Autodesk Inventor part; units mm, degrees
ref_plane "YZ Plane" through (0, 0, 0) normal (1, 0, 0) x (0, 1, 0)
ref_plane "XZ Plane" through (0, 0, 0) normal (0, 1, 0) x (-1, 0, 0)
ref_plane "XY Plane" through (0, 0, 0) normal (0, 0, 1) x (1, 0, 0)
sketch "Sketch1" plane through (0, 0, 0) normal (0, 0, 1) x (1, 0, 0)
  circle A0 centre (16.975, 77.075) radius 1.621
  circle A1 centre (0, 60.25) radius 1.621
  circle A2 centre (-16.975, 77.075) radius 1.621
  line L0 (-19.5, 89.5) -> (-19.5, 43.5)
  line L1 (-19.5, 43.5) -> (-13.8, 43.5)
  line L2 (-13.8, 43.5) -> (-13.8, 49.1)
  arc A3 (-10.8, 52.1) -> (-13.8, 49.1) centre (-10.8, 49.1) ccw
  line L3 (-10.8, 52.1) -> (10.8, 52.1)
  arc A4 (13.8, 49.1) -> (10.8, 52.1) centre (10.8, 49.1) ccw
  line L4 (13.8, 49.1) -> (13.8, 43.5)
  line L5 (13.8, 43.5) -> (19.5, 43.5)
  line L6 (19.5, 43.5) -> (19.5, 89.5)
  line L7 (19.5, 89.5) -> (-19.5, 89.5)
  circle A5 centre (-17, 46.5) radius 1.25
  circle A6 centre (17, 46.5) radius 1.25
  circle A7 centre (17, 86.5) radius 1.25
  circle A8 centre (-17, 86.5) radius 1.25
  line L8 (-19.5, 89.5) -> (19.5, 89.5)
  line L9 (19.5, 89.5) -> (19.5, 43.5)
  line L10 (19.5, 43.5) -> (-19.5, 43.5)
  line L11 (-19.5, 43.5) -> (-19.5, 89.5)
  point P0 (0, 0)
  point P1 (-13.8, 43.5)
  point P2 (13.8, 43.5)
extrude "Extrusion1" add sketch "Sketch1" along normal blind 4 contours A0 | A1 | A2 | L7 L6 L5 L4 A4 L3 A3 L2 L1 L0 | L2 A3 L3 A4 L4 L10 | A5 | A6 | A7 | A8
sketch "Sketch2" plane through (0, 0, 4) normal (0, 0, 1) x (1, 0, 0)
  circle A0 centre (16.975, 77.075) radius 1.621
  circle A1 centre (0, 60.25) radius 1.621
  circle A2 centre (-16.975, 77.075) radius 1.621
  line L0 (-19.5, 89.5) -> (-19.5, 43.5)
  line L1 (-19.5, 43.5) -> (-13.8, 43.5)
  line L2 (-13.8, 43.5) -> (-13.8, 49.1)
  arc A3 (-10.8, 52.1) -> (-13.8, 49.1) centre (-10.8, 49.1) ccw
  line L3 (-10.8, 52.1) -> (10.8, 52.1)
  arc A4 (13.8, 49.1) -> (10.8, 52.1) centre (10.8, 49.1) ccw
  line L4 (13.8, 49.1) -> (13.8, 43.5)
  line L5 (13.8, 43.5) -> (19.5, 43.5)
  line L6 (19.5, 43.5) -> (19.5, 89.5)
  line L7 (19.5, 89.5) -> (-19.5, 89.5)
  circle A5 centre (-17, 46.5) radius 1.25
  circle A6 centre (17, 46.5) radius 1.25
  circle A7 centre (17, 86.5) radius 1.25
  circle A8 centre (-17, 86.5) radius 1.25
  point P0 (0, 0)
hole "Hole1" at (-16.975, 77.075, 4) at (16.975, 77.075, 4) at (0, 60.25, 4) direction (0, 0, -1) diameter 4.8 depth 5 countersink diameter 9.4 countersink angle 90
sketch "Sketch3" plane through (0, 0, 0) normal (0, 0, -1) x (-1, 0, 0)
  line L0 (-19.5, 81.0391) -> (-19.5, 89.5)
  line L1 (-19.5, 89.5) -> (19.5, 89.5)
  line L2 (19.5, 89.5) -> (19.5, 81.0391)
  line L3 (19.5, 43.5) -> (-19.5, 43.5)
  line L4 (-19.5, 89.5) -> (19.5, 89.5)
  line L5 (19.5, 89.5) -> (26.5, 89.5)
  line L6 (26.5, 89.5) -> (26.5, 82.5)
  line L7 (26.5, 82.5) -> (19.5, 82.5)
  line L8 (19.5, 82.5) -> (19.5, 89.5)
  line L9 (-19.5, 89.5) -> (-26.5, 89.5)
  line L10 (-26.5, 89.5) -> (-26.5, 82.5)
  line L11 (-26.5, 82.5) -> (-19.5, 82.5)
  line L12 (-19.5, 82.5) -> (-19.5, 89.5)
  line L13 (19.5, 43.5) -> (-19.5, 43.5)
  line L14 (19.5, 43.5) -> (26.5, 43.5)
  line L15 (26.5, 43.5) -> (26.5, 50.5)
  line L16 (26.5, 50.5) -> (19.5, 50.5)
  line L17 (19.5, 50.5) -> (19.5, 43.5)
  line L18 (-19.5, 50.5) -> (-26.5, 50.5)
  line L19 (-26.5, 50.5) -> (-26.5, 43.5)
  line L20 (-26.5, 43.5) -> (-19.5, 43.5)
  line L21 (-19.5, 43.5) -> (-19.5, 50.5)
  arc A0 (-19.5, 73.1109) -> (-19.5, 81.0391) centre (-16.975, 77.075) ccw
  arc A1 (19.5, 81.0391) -> (19.5, 73.1109) centre (16.975, 77.075) ccw
  line L22 (19.5, 73.1109) -> (19.5, 43.5)
  line L23 (-19.5, 43.5) -> (-19.5, 73.1109)
  point P0 (0, 0)
  point P1 (-19.5, 82.5)
  point P2 (19.5, 82.5)
  dimension "d9" = 7
  dimension "d10" = 7
  dimension "d11" = 7
  dimension "d12" = 7
  dimension "d15" = 7
  dimension "d16" = 7
  dimension "d17" = 7
  dimension "d18" = 7
  dimension "d19" = 0
extrude "Extrusion2" add sketch "Sketch3" against normal up to surface (4 mm away) contours L11 L10 L9 L0 | L21 L20 L19 L18 | L5 L6 L7 L2 | L17 L16 L15 L14
sketch "Sketch4" plane through (0, 0, 0) normal (0, 0, -1) x (-1, 0, 0)
  line L0 (26.5, 43.5) -> (-26.5, 43.5)
  line L1 (26.5, 43.5) -> (26.5, 50.5)
  line L2 (26.5, 50.5) -> (19.5, 50.5)
  line L3 (19.5, 82.5) -> (19.5, 50.5)
  line L4 (19.5, 82.5) -> (26.5, 82.5)
  line L5 (26.5, 82.5) -> (26.5, 89.5)
  line L6 (26.5, 89.5) -> (-26.5, 89.5)
  line L7 (-26.5, 89.5) -> (-26.5, 82.5)
  line L8 (-26.5, 82.5) -> (-19.5, 82.5)
  line L9 (-19.5, 50.5) -> (-19.5, 82.5)
  line L10 (-19.5, 50.5) -> (-26.5, 50.5)
  line L11 (-26.5, 50.5) -> (-26.5, 43.5)
  line L12 (26.5, 50.5) -> (19.5, 43.5)
  line L13 (19.5, 82.5) -> (19.5, 50.5)
  line L14 (26.5, 43.5) -> (19.5, 50.5)
  line L15 (-26.5, 50.5) -> (-26.5, 43.5)
  line L16 (-26.5, 50.5) -> (-19.5, 43.5)
  line L17 (-26.5, 43.5) -> (-19.5, 50.5)
  line L18 (26.5, 89.5) -> (19.5, 82.5)
  line L19 (26.5, 82.5) -> (19.5, 89.5)
  line L20 (-19.5, 50.5) -> (-19.5, 82.5)
  line L21 (-26.5, 89.5) -> (-19.5, 82.5)
  line L22 (-19.5, 82.5) -> (-26.5, 82.5)
  line L23 (-26.5, 82.5) -> (-19.5, 89.5)
  point P0 (0, 0)
  point P1 (19.5, 73.1109)
  point P2 (-19.5, 81.0391)
  point P3 (23, 47)
  point P4 (-23, 47)
  point P5 (-23, 86)
  point P6 (23, 86)
hole "Hole2" at (-23, 47, 0) at (23, 47, 0) at (23, 86, 0) at (-23, 86, 0) direction (0, 0, 1) diameter 3.6 depth 5
properties part number "vesc_holder"
Check sheet for the modelled part. Datum: model origin and axes. Units: mm. A direction names the side the tool comes from. Give positions to 0.01 mm unless a question says otherwise; leave off trailing zeros. Order: outer loops, then holes, each group sorted by start corner. A loop starts at its lowest first (then second) coordinate and runs counter-clockwise, first axis right, second up. Notation, with made-up numbers: (75.5, 5.5) - (93.5, 5.5) arc R22 ccw to (93.5, 42.5) - close; hole circle Ø11 at (30.5, 55.5). An arc over 180 degrees is marked (long way). Answer as CSV lines item,"result".
1. Section check A-A (y = 86). Record the boundary of the cut face in (x, z).
Result sheet:
outline,"(-26.5, 0) - (-24.8, 0) - (-24.8, 4) - (-26.5, 4) - close; (-21.2, 0) - (21.2, 0) - (21.2, 4) - (-21.2, 4) - close; (24.8, 0) - (26.5, 0) - (26.5, 4) - (24.8, 4) - close"
2. Go/stop test with flat-tipped pins: P1, Ø1.2, axis at y = 66, z = 1.5, coming from the -X side; P2, Ø2, axis at y = 65.5, z = 0.5, coming from the +X side. Record where each tip stops, or that it passes through.
Result sheet:
P1,"x = -19.5"
P2,"x = 19.5"
3. Section check D-D (z = 0.75). Record the boundary of the cut face in (x, y) (3 decimals).
Result sheet:
outline,"(-26.5, 43.5) - (26.5, 43.5) - (26.5, 50.5) - (19.5, 50.5) - (19.5, 82.5) - (26.5, 82.5) - (26.5, 89.5) - (-26.5, 89.5) - (-26.5, 82.5) - (-19.5, 82.5) - (-19.5, 50.5) - (-26.5, 50.5) - close; hole circle Ø3.6 at (-23, 47); hole circle Ø3.6 at (-23, 86); hole circle Ø4.8 at (-16.975, 77.075); hole circle Ø4.8 at (0, 60.25); hole circle Ø4.8 at (16.975, 77.075); hole circle Ø3.6 at (23, 47); hole circle Ø3.6 at (23, 86)"
4. Section check B-B (x = 0). Record the boundary of the cut face in (y, z).
Result sheet:
outline,"(43.5, 0) - (57.85, 0) - (57.85, 1.7) - (55.55, 4) - (43.5, 4) - close; (62.65, 0) - (89.5, 0) - (89.5, 4) - (64.95, 4) - (62.65, 1.7) - close"
5. Scan lines: probe 1 along Y at (x, z) = (23, 2.75); probe 2 along Y at (x, z) = (24.5, 3.1); probe 3 along X at (y, z) = (85, 3.2). Record each from-to range of solid material in increasing order. Write a range as from..to.
Result sheet:
probe 1,"43.5..45.2, 48.8..50.5, 82.5..84.2, 87.8..89.5"
probe 2,"43.5..46.01, 47.99..50.5, 82.5..85.01, 86.99..89.5"
probe 3,"-26.5..-24.5, -21.5..21.5, 24.5..26.5"
6. Mould release check, pull along Y, two halves, no side actions. Record for faces 4 (the face through (0, 89.5, 2)), 5 (the face through (23, 82.5, 2)), 6 (the face through (26.5, 86, 2)): released by +Y, released by -Y, zero draft, split by the parting line, or undercut.
Result sheet:
face 4,"released by +Y"
face 5,"undercut"
face 6,"zero draft"
7. Section check C-C (x = -23). Record the boundary of the cut face in (y, z), then the cut area to 3 significant figures.
Result sheet:
outline,"(43.5, 0) - (45.2, 0) - (45.2, 4) - (43.5, 4) - close; (48.8, 0) - (50.5, 0) - (50.5, 4) - (48.8, 4) - close; (82.5, 0) - (84.2, 0) - (84.2, 4) - (82.5, 4) - close; (87.8, 0) - (89.5, 0) - (89.5, 4) - (87.8, 4) - close"
area,"27.2 mm²"
8. Tool access check on faces 1 (the face through (-19.5, 67, 2)), 2 (the face through (23, 50.5, 2)), 3 (the face through (14.492, 77.626, 1.844)). Record the directions out of +Z, -Z, +X, -X, +Y, -Y that give a thin tool (end or side, any length) a straight path to the whole face; none if there is none.
Result sheet:
face 1,"+Z, -Z, -X"
face 2,"+Z, -Z, +X"
face 3,"+Z"
